Geometry: see drawing. Coordinates: mm, zero at the bounding-box minimum. A direction names the side the tool comes from. Give positions to 0.01 mm unless a question says otherwise; leave off trailing zeros. Write each loop counter-clockwise with the first axis right and the second up, starting at its lowest first coordinate (ties: lowest second). Pieces come first, ordered by that corner, then holes.
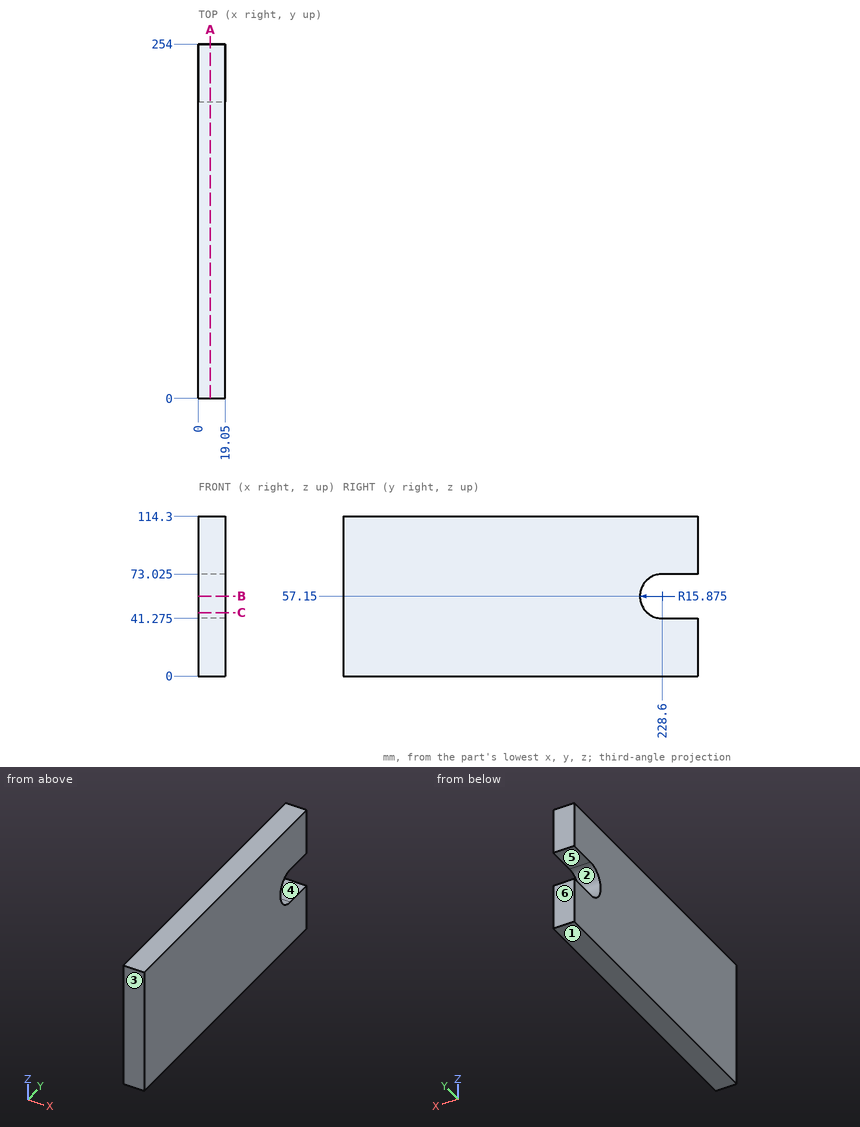
1. Pin query (flat end, axial travel): P1, Ø8, axis at x = 9, z = 66, coming from the +Y side. Return the tip coordinate at first contact, or that it passes through.
2. Section query C-C (z = 45.5). Return loops of the section in (x, y).
3. Pull-direction query (Z, two-part tool) for the marked faces 1, 2, 3 and 4; classes: pulls with the +Z half, pulls with the -Z half, needs draft (parallel to the pull), parting line crosses it, or undercut.
4. Line query: probe 1 along Z at (x, y) = (11.5, 232) (3 decimals); probe 2 along Z at (x, y) = (3.25, 219). Output: solid intervals per line, ascending.
5. Section query B-B (z = 57.15). Return loops of the section in (x, y) (3 decimals).
6. Section query A-A (x = 8.5). Return loops of the section in (y, z) (3 decimals).
7. Access query for the marked faces 5 and 6. Directions: +Z, -Z, +X, -X, +Y, -Y. A direction counts if a zero-diameter tool reaches every point of the face in a straight line with its end or side. Return the directions, or none.
The answers:
1. P1: stops at y = 219.28
2. outline: (0, 0) - (19.05, 0) - (19.05, 217.82) - (0, 217.82) - close
3. face 1: pulls with the -Z half
3. face 2: undercut
3. face 3: needs draft
3. face 4: undercut
4. probe 1: z = 0 to 41.275, 73.025 to 114.3
4. probe 2: z = 0 to 44.51, 69.79 to 114.3
5. outline: (0, 0) - (19.05, 0) - (19.05, 212.725) - (0, 212.725) - close
6. outline: (0, 0) - (254, 0) - (254, 41.275) - (228.6, 41.275) arc R15.875 cw to (228.6, 73.025) - (254, 73.025) - (254, 114.3) - (0, 114.3) - close
7. face 5: +X, -X, +Y
7. face 6: +Z, -Z, +X, -X, +Y
